The model under review builds one solid part; all positions refer to its coordinate system, in mm. A direction names the side the tool comes from. Round coordinates to 2 decimals unless told otherwise and drop trailing zeros. Order: outer loops, then holes, each group sorted by start corner. A loop starts at its lowest first (then second) coordinate and runs counter-clockwise, first axis right, second up. Notation, with made-up numbers: M -23.5,11.25 L -5.5,11.25 A19 ccw -5.5,19.25 Z; hole C 36,84.25 d4. An arc over 180 degrees is marked long. One line per item, written item: value. Start each with the question number.
Autodesk Inventor part; units mm, degrees
ref_plane "YZ Plane" through (0, 0, 0) normal (1, 0, 0) x (0, 1, 0)
ref_plane "XZ Plane" through (0, 0, 0) normal (0, 1, 0) x (-1, 0, 0)
ref_plane "XY Plane" through (0, 0, 0) normal (0, 0, 1) x (1, 0, 0)
sketch "Sketch1" plane through (0, 0, 0) normal (0, 0, 1) x (1, 0, 0)
  line L0 (43.65, -17.5) -> (-43.65, -17.5)
  line L1 (-50, -11.15) -> (-50, 11.15)
  line L2 (-43.65, 17.5) -> (43.65, 17.5)
  line L3 (50, 11.15) -> (50, -11.15)
  line L4 (50, -17.5) -> (-50, 17.5) construction
  line L5 (-50, -17.5) -> (50, 17.5) construction
  line L6 (0, 51.2558) -> (0, -45.9758)
  circle A0 centre (-40, 0) radius 5.1
  line L7 (-83.6339, 0) -> (65.0593, 0)
  circle A1 centre (40, 0) radius 5.1
  circle A2 centre (0, 0) radius 5.1
  arc A3 (-43.65, 17.5) -> (-50, 11.15) centre (-43.65, 11.15) ccw
  arc A4 (-50, -11.15) -> (-43.65, -17.5) centre (-43.65, -11.15) ccw
  arc A5 (43.65, -17.5) -> (50, -11.15) centre (43.65, -11.15) ccw
  arc A6 (50, 11.15) -> (43.65, 17.5) centre (43.65, 11.15) ccw
  line L8 (-14.905, -13) -> (-20.655, -13)
  line L9 (-23.83, -9.825) -> (-23.83, 9.825)
  line L10 (-20.655, 13) -> (-14.905, 13)
  line L11 (-11.73, 9.825) -> (-11.73, -9.825)
  line L12 (-11.73, -13) -> (-23.83, 13) construction
  line L13 (-23.83, -13) -> (-11.73, 13) construction
  line L14 (14.905, -13) -> (20.655, -13)
  line L15 (23.83, -9.825) -> (23.83, 9.825)
  line L16 (20.655, 13) -> (14.905, 13)
  line L17 (11.73, 9.825) -> (11.73, -9.825)
  line L18 (11.73, -13) -> (23.83, 13) construction
  line L19 (23.83, -13) -> (11.73, 13) construction
  arc A7 (-20.655, 13) -> (-23.83, 9.825) centre (-20.655, 9.825) ccw
  arc A8 (-11.73, 9.825) -> (-14.905, 13) centre (-14.905, 9.825) ccw
  arc A9 (-14.905, -13) -> (-11.73, -9.825) centre (-14.905, -9.825) ccw
  arc A10 (-23.83, -9.825) -> (-20.655, -13) centre (-20.655, -9.825) ccw
  arc A11 (11.73, -9.825) -> (14.905, -13) centre (14.905, -9.825) ccw
  arc A12 (20.655, -13) -> (23.83, -9.825) centre (20.655, -9.825) ccw
  arc A13 (23.83, 9.825) -> (20.655, 13) centre (20.655, 9.825) ccw
  arc A14 (14.905, 13) -> (11.73, 9.825) centre (14.905, 9.825) ccw
  point P0 (0, 0)
  point P1 (0, 0)
  point P2 (-17.78, 0)
  point P3 (17.78, 0)
  dimension "d0" = 100
  dimension "d1" = 35
  dimension "d2" = 80
  dimension "d3" = 10.2
  dimension "d6" = 10.2
  dimension "d7" = 6.35
  dimension "d8" = 26
  dimension "d9" = 12.1
  dimension "d10" = 3.175
  dimension "d11" = 35.56
extrude "Extrusion1" add sketch "Sketch1" along normal blind 6.35 contours L0 L6 A2 L7 L17 A11 L14 A12 L15 A1 L3 A5 | L0 A4 L1 L7 A0 L9 A10 L8 A9 L11 A2 L6 | L7 A1 L15 A13 L16 A14 L17 A2 L6 L2 A6 L3 | L7 L11 A8 L10 A7 L9 A0 L1 A3 L2 L6 A2
equation "\"d6\" = d3"
properties part number "Vertical_Lead_Screw_E-stop_Plate"
Item 1: Consider section D-D, the plane y = 0. Give the boundary of the cut face in (x, z), then the cut area to 3 significant figures.
Item 2: Wall thickness on L1, parallel to X at y = -6, z = 4.25; L2, parallel to X at y = 0, z = 4.5; L3, parallel to Y at x = 40, z = 4.5: over which ranges is each line inside the solid? List them lowest first.
Item 3: Consider section C-C, the plane z = 1. Give the boundary of the cut face in (x, y) (3 decimals).
Item 4: Machinability: for faces 1 (the flat face through (18, 13, 3)), 2 (the cylindrical face through (48.09, 15.69, 3.13)), which of the approach directions +Z, -Z, +X, -X, +Y, -Y give a long, thin tool a straight path to every point of the face, cutting with its end or side? Answer none if there is none.
Item 5: Consider section B-B, the plane x = 0. Give the boundary of the cut face in (y, z).
Item 6: Consider section A-A, the plane y = -8. Give the boundary of the cut face in (x, z).
Item 7: Clearance check with a flat-ended pin moving along its axis: P1, Ø8, axis at x = -40, y = 0, coming from the +Z side. State where the tip first meets the part, or that it passes through.
Item 8: The part is to be moulded in two halves that separate along X. For faces 3 (the flat face through (-50, 0, 3)), 4 (the flat face through (-1, 8, 6.35)), 5 (the flat face through (-18, 13, 3)), say which applies: pulls with the +X half, pulls with the -X half, needs draft (parallel to the pull), parting line crosses it, or undercut.
Computed:
1. outline: M -50,0 L -45.1,0 L -45.1,6.35 L -50,6.35 Z; M -34.9,0 L -23.83,0 L -23.83,6.35 L -34.9,6.35 Z; M -11.73,0 L -5.1,0 L -5.1,6.35 L -11.73,6.35 Z; M 5.1,0 L 11.73,0 L 11.73,6.35 L 5.1,6.35 Z; M 23.83,0 L 34.9,0 L 34.9,6.35 L 23.83,6.35 Z; M 45.1,0 L 50,0 L 50,6.35 L 45.1,6.35 Z
1. area: 287 mm^2
2. L1: x = -50 to -23.83, -11.73 to 11.73, 23.83 to 50
2. L2: x = -50 to -45.1, -34.9 to -23.83, -11.73 to -5.1, 5.1 to 11.73, 23.83 to 34.9, 45.1 to 50
2. L3: y = -17.5 to -5.1, 5.1 to 17.5
3. outline: M -50,-11.15 A6.35 ccw -43.65,-17.5 L 43.65,-17.5 A6.35 ccw 50,-11.15 L 50,11.15 A6.35 ccw 43.65,17.5 L -43.65,17.5 A6.35 ccw -50,11.15 Z; hole C -40,0 d10.2; hole M -23.83,-9.825 A3.175 ccw -20.655,-13 L -14.905,-13 A3.175 ccw -11.73,-9.825 L -11.73,9.825 A3.175 ccw -14.905,13 L -20.655,13 A3.175 ccw -23.83,9.825 Z; hole C 0,0 d10.2; hole M 11.73,-9.825 A3.175 ccw 14.905,-13 L 20.655,-13 A3.175 ccw 23.83,-9.825 L 23.83,9.825 A3.175 ccw 20.655,13 L 14.905,13 A3.175 ccw 11.73,9.825 Z; hole C 40,0 d10.2
4. face 1: +Z, -Z
4. face 2: +Z, -Z, +X, +Y
5. outline: M -17.5,0 L -5.1,0 L -5.1,6.35 L -17.5,6.35 Z; M 5.1,0 L 17.5,0 L 17.5,6.35 L 5.1,6.35 Z
6. outline: M -50,0 L -23.83,0 L -23.83,6.35 L -50,6.35 Z; M -11.73,0 L 11.73,0 L 11.73,6.35 L -11.73,6.35 Z; M 23.83,0 L 50,0 L 50,6.35 L 23.83,6.35 Z
7. P1: passes through
8. face 3: pulls with the -X half
8. face 4: needs draft
8. face 5: undercut
